```python
from build123d import *

# Parameters (mm, degrees)
SKETCH_1_W          = 96
SKETCH_1_H          = 57
EXTRUDE_1_DEPTH     = 36
SKETCH_2_W          = 8
SKETCH_2_H          = 22
CUT_EXTRUDE_1_DEPTH = 54
CUT_EXTRUDE_2_DEPTH = 54
SKETCH_5_W          = 68
SKETCH_5_H          = 6.822468225
EXTRUDE_2_DEPTH     = 14


with BuildPart() as part:
    # 스케치1 → 보스-돌출1 (new body)
    with BuildSketch(Plane.XY):
        Rectangle(SKETCH_1_W, SKETCH_1_H)
    extrude(amount=EXTRUDE_1_DEPTH)

    # 스케치2 → 컷-돌출1 (cut)
    with BuildSketch(Plane(origin=(0, 28.5, 0), x_dir=(1, 0, 0), z_dir=(0, 1, 0))):
        with Locations((-44, -25)):
            Rectangle(SKETCH_2_W, SKETCH_2_H)
        with Locations((44, -25)):
            Rectangle(SKETCH_2_W, SKETCH_2_H)
    extrude(amount=-CUT_EXTRUDE_1_DEPTH, mode=Mode.SUBTRACT)

    # 스케치4 → 컷-돌출2 (cut)
    with BuildSketch(Plane(origin=(0, -25.5, 0), x_dir=(1, 0, 0), z_dir=(0, 1, 0))):
        with BuildLine():
            Line((48, -26), (43.25, -26))
            ThreePointArc((43.25, -26), (41, -23.75), (43.25, -21.5))
            Line((43.25, -21.5), (48, -21.5))
            Line((48, -21.5), (48, -26))
        make_face()
    cut_extrude_2 = extrude(amount=-CUT_EXTRUDE_2_DEPTH, mode=Mode.SUBTRACT)

    # 대칭 복사1: 컷-돌출2 across plane
    add(cut_extrude_2.mirror(Plane(origin=(0, 0, 0), x_dir=(0, 0, 1), z_dir=(1, 0, 0))), mode=Mode.SUBTRACT)

    # 스케치5 → 보스-돌출2 (add)
    with BuildSketch(Plane(origin=(0, 28.5, 0), x_dir=(1, 0, 0), z_dir=(0, 1, 0))):
        with Locations((0, -32.588765888)):
            Rectangle(SKETCH_5_W, SKETCH_5_H)
    extrude(amount=EXTRUDE_2_DEPTH)


solid = part.part
```
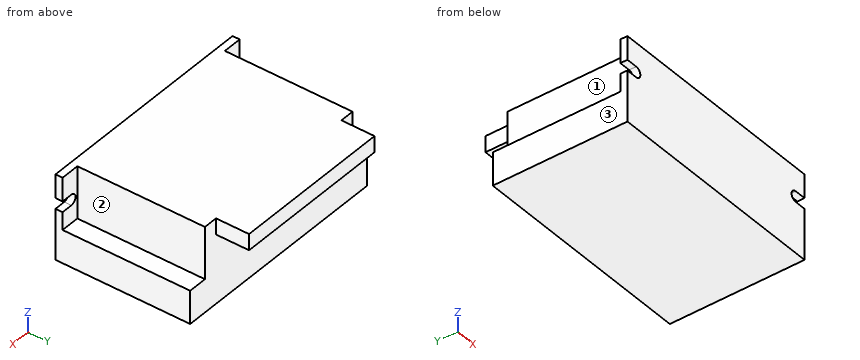
CAD build for the part. Positions are in the model's coordinates, mm. Face numbers are marked on the shaded views. A direction names the side the tool comes from. Round coordinates to 2 decimals unless told otherwise and drop trailing zeros. Order: outer loops, then holes, each group sorted by start corner. A loop starts at its lowest first (then second) coordinate and runs counter-clockwise, first axis right, second up.
Item 1: Saw through at D-D on z = 4. Write the cut outline in (x, y).
Item 2: Probe line 1 along Y through (x, z) = (-24, 29); line 2 along X through (y, z) = (37, 30.5); line 3 along X through (y, z) = (-17, 29.5). List the from-to ranges inside material, lowest first.
Item 3: Saw through at C-C on x = -18.5. Write the cut outline in (y, z), then the cut area to 3 significant figures.
Item 4: Saw through at B-B on y = -2. Write the cut outline in (x, z), then the cut area to 3 significant figures.
Item 5: Pin check, flat tips, straight feed: pin 1 (4 mm diameter, centred on x = -44.5, y = 4, fed in from +Z); pin 2 (5.5 mm diameter, centred on y = 34.5, z = 32.5, fed in from -X); pin 3 (5 mm diameter, centred on y = -14.5, z = 17, fed in from +X). Stop position of each tip, or through.
Item 6: Saw through at A-A on z = 23.75. Write the cut outline in (x, y).
Item 7: Tool access for the marked faces 1, 2 and 3: list every direction of +Z, -Z, +X, -X, +Y, -Y with a clear straight run to the whole face (end or side of a thin tool).
Reported:
1. outline: (-48, -28.5) - (48, -28.5) - (48, 28.5) - (-48, 28.5) - close
2. line 1: y = -28.5 to 28.5
2. line 2: x = -34 to 34
2. line 3: x = -40 to 40
3. outline: (-28.5, 0) - (28.5, 0) - (28.5, 29.18) - (42.5, 29.18) - (42.5, 36) - (-28.5, 36) - close
3. area: 2,150 mm2
4. outline: (-48, 0) - (48, 0) - (48, 14) - (40, 14) - (40, 36) - (-40, 36) - (-40, 14) - (-48, 14) - close
4. area: 3,100 mm2
5. pin 1: stops at z = 14
5. pin 2: stops at x = -34
5. pin 3: stops at x = 40
6. outline: (-41, -28.5) - (41, -28.5) - (41, -25.5) - (40, -25.5) - (40, 28.5) - (-40, 28.5) - (-40, -25.5) - (-41, -25.5) - close
7. face 1: +Z, -X, +Y
7. face 2: +Z, +X, +Y
7. face 3: +Z, -Z, -X, +Y, -Y
